```python
from build123d import *

# Parameters (mm, degrees)
SKETCH1_W           = 50
SKETCH1_H           = 80
BOSS_EXTRUDE1_DEPTH = 45
SKETCH5_W           = 42
SKETCH5_H           = 42
CUT_EXTRUDE1_DEPTH  = 40
SKETCH6_R           = 1.5
CUT_EXTRUDE2_DEPTH  = 40
SKETCH7_W           = 15
SKETCH7_H           = 41.689626702
CUT_EXTRUDE3_DEPTH  = 10
SKETCH8_R           = 11
CUT_EXTRUDE4_DEPTH  = 2
SKETCH9_R           = 2
CUT_EXTRUDE5_DEPTH  = 10
SKETCH2_R           = 2.5
CUT_EXTRUDE6_DEPTH  = 10
SKETCH10_R          = 7.5
CUT_EXTRUDE7_DEPTH  = 48


with BuildPart() as part:
    # Sketch1 → Boss-Extrude1 (new body)
    with BuildSketch(Plane.XY):
        Rectangle(SKETCH1_W, SKETCH1_H)
    extrude(amount=BOSS_EXTRUDE1_DEPTH)

    # Sketch5 → Cut-Extrude1 (cut)
    with BuildSketch(Plane.XY.offset(45)):
        with Locations((0, -15)):
            Rectangle(SKETCH5_W, SKETCH5_H)
    extrude(amount=-CUT_EXTRUDE1_DEPTH, mode=Mode.SUBTRACT)

    # Sketch6 → Cut-Extrude2 (cut)
    with BuildSketch(Plane.XY.offset(5)):
        with Locations((15.5, -30.5)):
            Circle(SKETCH6_R)
        with Locations((15.5, 0.5)):
            Circle(SKETCH6_R)
        with Locations((-15.5, -30.5)):
            Circle(SKETCH6_R)
        with Locations((-15.5, 0.5)):
            Circle(SKETCH6_R)
    extrude(amount=-CUT_EXTRUDE2_DEPTH, mode=Mode.SUBTRACT)

    # Sketch7 → Cut-Extrude3 (cut)
    with BuildSketch(Plane.XY.offset(45)):
        with Locations((0, -40)):
            Rectangle(SKETCH7_W, SKETCH7_H)
    extrude(amount=-CUT_EXTRUDE3_DEPTH, mode=Mode.SUBTRACT)

    # Sketch8 → Cut-Extrude4 (cut)
    with BuildSketch(Plane.XY.offset(5)):
        with Locations((0, -15)):
            Circle(SKETCH8_R)
    extrude(amount=-CUT_EXTRUDE4_DEPTH, mode=Mode.SUBTRACT)

    # Sketch9 → Cut-Extrude5 (cut)
    with BuildSketch(Plane.XY.offset(3)):
        with Locations((0, -15)):
            Circle(SKETCH9_R)
    extrude(amount=-CUT_EXTRUDE5_DEPTH, mode=Mode.SUBTRACT)

    # Sketch2 → Cut-Extrude6 (cut)
    with BuildSketch(Plane(origin=(0, 0, 0), x_dir=(-1, 0, 0), z_dir=(0, 0, -1))):
        with Locations((0, 20)):
            Circle(SKETCH2_R)
    extrude(amount=-CUT_EXTRUDE6_DEPTH, mode=Mode.SUBTRACT)

    # Sketch10 → Cut-Extrude7 (cut)
    with BuildSketch(Plane(origin=(0, 0, 0), x_dir=(-1, 0, 0), z_dir=(0, 0, -1))):
        with Locations((0, 20)):
            Circle(SKETCH10_R)
    extrude(amount=-CUT_EXTRUDE7_DEPTH, mode=Mode.SUBTRACT)


solid = part.part
```
The listing builds one solid part. Answer for the finished solid, in the listing's coordinates (mm). A direction names the side the tool comes from. Round coordinates to 2 decimals unless told otherwise and drop trailing zeros. Loops run counter-clockwise (first coordinate to the right, second up) from the corner with the lowest first, then second, coordinate; pieces in that order, holes last. Notation, with made-up numbers: (-11, -33.75) - (40, -33.75) arc R22 ccw to (40, -13.75) - close; hole circle Ø4 at (8.25, -26). An arc over 180 degrees is marked (long way). Return JSON: item names as keys, results as strings. Group by question number.
1. The part is cut by section D-D on y = 0.5. Determine the outline of the cut face in (x, z).
2. Each of these flat-tipped pins is pushed along its axis until it touches: P1, Ø10, axis at x = -1.5, y = -7, coming from the +Z side; P2, Ø2, axis at x = -0.5, y = -38.5, coming from the +Z side; P3, Ø13.5, axis at x = 0, y = 20, coming from the -Z side; P4, Ø12.5, axis at x = 1, y = -13.5, coming from the +Z side. Where does it stop, or does it pass through?
3. The part is cut by section C-C on z = 33. Determine the outline of the cut face in (x, y).
4. The part is cut by section A-A on x = 15.5. Determine the outline of the cut face in (y, z).
5. The part is cut by section B-B on y = -15. Determine the outline of the cut face in (x, z), then the cut area to 3 significant figures.
6. The mould has two halves that part along Y. Classify faces 4 (the flat face through (0, 40, 22)), 5 (the flat face through (-7.5, -38, 40)), 6 (the flat face through (-21, -15, 25)): pulls with the +Y half, pulls with the -Y half, needs draft (parallel to the pull), parting line crosses it, or undercut.
7. Which of the six approach directions +Z, -Z, +X, -X, +Y, -Y give full straight-line access (tool end or side, diameter ignored) to faces 1 (the cylindrical face through (-17, 0.57, 2.54)), 2 (the flat face through (-10, -24, 5)), 3 (the flat face through (0, -38, 35))?
8. Consider probe 1 along Y at (x, z) = (0, 1.35); probe 2 along Y at (x, z) = (-15.5, 1.2); probe 3 along Y at (x, z) = (13, 11). Determine where each line is inside the solid, lowest interval first.
Resolved:
{
 "1": {"outline": "(-25, 0) - (-17, 0) - (-17, 5) - (-21, 5) - (-21, 45) - (-25, 45) - close; (-14, 0) - (14, 0) - (14, 5) - (-14, 5) - close; (17, 0) - (25, 0) - (25, 45) - (21, 45) - (21, 5) - (17, 5) - close"},
 "2": {"P1": "stops at z = 5", "P2": "stops at z = 35", "P3": "passes through", "P4": "stops at z = 3"},
 "3": {"outline": "(-25, -40) - (25, -40) - (25, 40) - (-25, 40) - close; hole (-21, -36) - (21, -36) - (21, 6) - (-21, 6) - close; hole circle Ø15 at (0, 20)"},
 "4": {"outline": "(-40, 0) - (-32, 0) - (-32, 5) - (-36, 5) - (-36, 45) - (-40, 45) - close; (-29, 0) - (-1, 0) - (-1, 5) - (-29, 5) - close; (2, 0) - (40, 0) - (40, 45) - (6, 45) - (6, 5) - (2, 5) - close"},
 "5": {"outline": "(-25, 0) - (-2, 0) - (-2, 3) - (-11, 3) - (-11, 5) - (-21, 5) - (-21, 45) - (-25, 45) - close; (2, 0) - (25, 0) - (25, 45) - (21, 45) - (21, 5) - (11, 5) - (11, 3) - (2, 3) - close", "area": "514 mm²"},
 "6": {"face 4": "pulls with the +Y half", "face 5": "needs draft", "face 6": "undercut"},
 "7": {"face 1": "+Z, -Z", "face 2": "+Z", "face 3": "+Z, -Y"},
 "8": {"probe 1": "y = -40 to -17, -13 to 12.5, 27.5 to 40", "probe 2": "y = -40 to -32, -29 to -1, 2 to 40", "probe 3": "y = -40 to -36, 6 to 40"}
}
